from build123d import *

# Parameters (mm, degrees)
SKETCH1_R                = 3.81
BOSS_EXTRUDE1_DEPTH      = 10.922
CUT_EXTRUDE1_DEPTH       = 13.633787397
CUT_EXTRUDE2_DEPTH       = 10.922
BOSS_EXTRUDE2_REACH      = 14.179
BOSS_EXTRUDE2_END_RADIUS = 6.858
SKETCH4_W                = 4.064
SKETCH4_H                = 2.54
BOSS_EXTRUDE3_REACH      = 15.641
BOSS_EXTRUDE3_END_RADIUS = 4.064
FILLET1_R                = 0.762


with BuildPart() as part:
    # Sketch1 → Boss-Extrude1 (new, symmetric)
    with BuildSketch(Plane.XY):
        Circle(SKETCH1_R)
    extrude(amount=BOSS_EXTRUDE1_DEPTH, both=True)

    # Sketch2 → Cut-Extrude1 (cut, through all)
    with BuildSketch(Plane(origin=(0, 1.27, 0), x_dir=(1, 0, 0), z_dir=(0, 1, 0))):
        Polygon((-3.81, 3.683), (3.81, 3.683), (3.81, -3.937), (1.016, -3.937), (1.016, -0.762), (-1.016, -0.762), (-1.016, -3.937), (-3.81, -3.937), align=None)
    cut_extrude1 = extrude(amount=CUT_EXTRUDE1_DEPTH, mode=Mode.SUBTRACT)

    # Mirror1: Cut-Extrude1 across plane
    add(cut_extrude1.mirror(Plane.ZX), mode=Mode.SUBTRACT)

    # Sketch3 → Cut-Extrude2 (cut, symmetric)
    with BuildSketch(Plane(origin=(0, 0, 0), x_dir=(0, 0, -1), z_dir=(1, 0, 0))):
        with BuildLine():
            Line((5.207, -1.27), (5.207, 1.27))
            ThreePointArc((5.207, 1.27), (6.045841446, 2.108841446), (6.884682892, 1.27))
            Line((6.884682892, 1.27), (6.884682892, 0.635))
            Line((6.884682892, 0.635), (9.652, 0.635))
            Line((9.652, 0.635), (9.652, -3.81))
            Line((9.652, -3.81), (8.89, -3.81))
            Line((8.89, -3.81), (8.89, -0.635))
            Line((8.89, -0.635), (6.884682892, -0.635))
            Line((6.884682892, -0.635), (6.884682892, -1.27))
            ThreePointArc((6.884682892, -1.27), (6.045841446, -2.108841446), (5.207, -1.27))
        make_face()
    extrude(amount=CUT_EXTRUDE2_DEPTH, both=True, mode=Mode.SUBTRACT)

    # Boss-Extrude2: up to this cylinder (the profile starts inside it)
    boss_extrude2_end = Plane(origin=(0, 0, 2.54), z_dir=(0, 0, -1)) * Cylinder(BOSS_EXTRUDE2_END_RADIUS, 43.074, mode=Mode.PRIVATE)
    # Sketch4 → Boss-Extrude2 (add, up to the surface)
    with BuildSketch(Plane(origin=(0, 0, 0), x_dir=(0, 0, -1), z_dir=(1, 0, 0)), mode=Mode.PRIVATE) as boss_extrude2_sk1:
        with Locations((-2.54, 0)):
            Rectangle(SKETCH4_W, SKETCH4_H)
    boss_extrude2_tool1 = extrude(boss_extrude2_sk1.sketch, amount=BOSS_EXTRUDE2_REACH, mode=Mode.PRIVATE) & boss_extrude2_end
    add(boss_extrude2_tool1.solids().sort_by_distance((0, 0, 2.54))[0])

    # Boss-Extrude3: up to this cylinder (the profile starts inside it)
    boss_extrude3_end = Plane(origin=(0, 0, -8.128), z_dir=(0, 0, -1)) * Cylinder(BOSS_EXTRUDE3_END_RADIUS, 40.41, mode=Mode.PRIVATE)
    # Sketch5 → Boss-Extrude3 (add, up to the surface)
    with BuildSketch(Plane(origin=(0, 0.635, 0), x_dir=(1, 0, 0), z_dir=(0, 1, 0)), mode=Mode.PRIVATE) as boss_extrude3_sk1:
        with BuildLine():
            Line((-0.635, 8.636), (0.635, 8.636))
            ThreePointArc((0.635, 8.636), (1.143, 8.128), (0.635, 7.62))
            Line((0.635, 7.62), (-0.635, 7.62))
            ThreePointArc((-0.635, 7.62), (-1.143, 8.128), (-0.635, 8.636))
        make_face()
    boss_extrude3_tool1 = extrude(boss_extrude3_sk1.sketch, amount=BOSS_EXTRUDE3_REACH, mode=Mode.PRIVATE) & boss_extrude3_end
    boss_extrude3 = boss_extrude3_tool1.solids().sort_by_distance((0, 0.635, -8.128))[0]
    add(boss_extrude3)

    # Mirror2: Boss-Extrude3 across plane
    add(boss_extrude3.mirror(Plane.ZX))

    # Fillet1
    fillet1_edges = [part.edges().sort_by_distance(p)[0] for p in [
        (-3.81, 0, -10.922),
        (-3.81, 0, 10.922),
    ]]
    fillet(fillet1_edges, radius=FILLET1_R)


solid = part.part
Verification items for the finished model (mm, model axes). A direction names the side the tool comes from. Give positions to 0.01 mm unless a question says otherwise; leave off trailing zeros. Write each loop counter-clockwise with the first axis right and the second up, starting at its lowest first coordinate (ties: lowest second). Pieces come first, ordered by that corner, then holes.
(1) Cross-section at D-D (y = -2.75). State how many separate pieces and enclosed holes the cut face has, plus the area to 3 significant figures.
(2) Cross-section at A-A (y = 0). Enter the section's corners in (x, z).
(3) Cross-section at B-B (z = 1.5). Enter the section's corners in (x, y).
(4) Gauge pin test, flat ends, axial feed: pin 1 (4 mm diameter, centred on x = -0.5, z = 2, fed in from +Y); pin 2 (2 mm diameter, centred on y = 3, z = -8.5, fed in from -X); pin 3 (1.9 mm diameter, centred on x = -2, y = -3, fed in from -Z); pin 4 (3 mm diameter, centred on x = 4.5, z = -1.5, fed in from -Y). Record the tip position at first contact, or that the pin passes through.
(5) Access from +Z, -Z, +X, -X, +Y, -Y to the whole of each face (thin tool, end or side, straight path). Record for faces 1 (the face through (0, -2, -8.89)), 2 (the face through (0, 3, 0.762)), 3 (the face through (1.016, -2, 2)), 4 (the face through (2, 2, 3.937)).
(6) Cross-section at C-C (x = 4.75). Enter the section's corners in (y, z).
(7) Material ranges on line 1 (Z direction, x = -0.5, y = -2.25); line 2 (Z direction, x = -1.75, y = -1); line 3 (Z direction, x = -2.75, y = -1.75), recorded low to high.
(8) Mould release check, pull along Z, two halves, no side actions. Record for faces 5 (the face through (5, 0, 0.508)), 6 (the face through (0, 0.635, -8)), 7 (the face through (6.858, 0.018, 2.512)): +Z half, -Z half, draft (parallel to the pull), parting line (faces both ways), or undercut.
Worked out:
1. separate pieces: 3
1. enclosed holes: 0
1. area: 76.7 mm2
2. outline: (-3.81, -10.16) arc R0.76 ccw to (-3.05, -10.92) - (3.05, -10.92) arc R0.76 ccw to (3.81, -10.16) - (3.81, -9.65) - (-3.81, -9.65) - close; (-3.81, -5.21) - (3.81, -5.21) - (3.81, 0.51) - (6.86, 0.51) - (6.86, 4.57) - (3.81, 4.57) - (3.81, 10.16) arc R0.76 ccw to (3.05, 10.92) - (-3.05, 10.92) arc R0.76 ccw to (-3.81, 10.16) - close
3. outline: (-3.59, -1.27) - (-1.02, -1.27) - (-1.02, -3.67) arc R3.81 ccw to (1.02, -3.67) - (1.02, -1.27) - (6.74, -1.27) arc R6.86 ccw to (6.74, 1.27) - (1.02, 1.27) - (1.02, 3.67) arc R3.81 ccw to (-1.02, 3.67) - (-1.02, 1.27) - (-3.59, 1.27) arc R3.81 ccw to start
4. pin 1: stops at y = 3.81
4. pin 2: stops at x = -3.24
4. pin 3: stops at z = -10.92
4. pin 4: stops at y = -1.27
5. face 1: +X, -X, -Y
5. face 2: +X, -X, +Y
5. face 3: +X, -Y
5. face 4: +X, +Y
6. outline: (-1.27, 0.51) - (1.27, 0.51) - (1.27, 4.57) - (-1.27, 4.57) - close
7. line 1: z = -10.92 to -9.65, -8.89 to -3.68, 0.76 to 10.92
7. line 2: z = -10.92 to -9.65, -8.89 to -6.88, -5.21 to 10.92
7. line 3: z = -10.89 to -9.65, -8.89 to -6.73, -5.36 to -3.68, 3.94 to 10.89
8. face 5: -Z half
8. face 6: undercut
8. face 7: draft
